Geometry check sheet. Reference: the model listing, model coordinates, mm. A direction names the side the tool comes from. Give positions to 0.01 mm unless a question says otherwise; leave off trailing zeros. Write each loop counter-clockwise with the first axis right and the second up, starting at its lowest first coordinate (ties: lowest second). Pieces come first, ordered by that corner, then holes. Notation, with made-up numbers: M 82,77.5 L 116,77.5 A14 cw 116,91.5 Z; hole C -30.5,36 d7. An arc over 180 degrees is marked long. Write each question's results on one line, items separated by ' | '.
Autodesk Inventor part; units mm, degrees
ref_plane "YZ Plane" through (0, 0, 0) normal (1, 0, 0) x (0, 1, 0)
ref_plane "XZ Plane" through (0, 0, 0) normal (0, 1, 0) x (-1, 0, 0)
ref_plane "XY Plane" through (0, 0, 0) normal (0, 0, 1) x (1, 0, 0)
sketch "Sketch2" plane through (0, 0, 0) normal (0, 0, 1) x (1, 0, 0)
  line L0 (1.5, 7.5) -> (1.5, 10.5)
  line L1 (1.5, 10.5) -> (3, 10.5)
  line L2 (3, 10.5) -> (3, 12.5)
  line L3 (3, 12.5) -> (5.75, 12.5)
  line L4 (5.75, 12.5) -> (10, 7.5)
  line L5 (10, 7.5) -> (10, 0)
  line L6 (1.5, 7.5) -> (5.75, 7.5)
  line L7 (5.75, 7.5) -> (5.75, 0)
  line L8 (5.75, 0) -> (10, 0)
  line L9 (0, 0) -> (0, 19.425)
  dimension "d0" = 6
  dimension "d1" = 3
  dimension "d2" = 11.5
  dimension "d3" = 20
  dimension "d4" = 7.5
  dimension "d5" = 3
  dimension "d6" = 2
revolve "Revolution1" add sketch "Sketch2" angle 360 about axis through (0, 0, 0) along (0, 1, 0)
sketch "Sketch3" plane through (0, 12.5, 0) normal (0, 1, 0) x (1, 0, 0)
  point P0 (0, 0)
  point P1 (0, 7.75)
  dimension "d8" = 7.75
hole "Hole1" at (0, 12.5, -7.75) direction (0, -1, 0) diameter 2.9 end through all counterbore diameter 5.5 counterbore depth 3.5
pattern_circular "Circular Pattern1" count 3 over 360 about axis through (0, -10, 0) along (0, 1, 0) of "Hole1"
properties part number "902-4250 magnet hold"
Q1. Depth check by flat-ended pin: P1, Ø3, axis at y = 4, z = 7.5, coming from the +X side; P2, Ø1.5, axis at y = 2, z = -6, coming from the -X side; P3, Ø2, axis at x = -7, y = 10.5, coming from the +Z side. Enter the tip coordinate at first touch or a pass-through.
Answer key:
P1: stops at x = 8 | P2: stops at x = -8.51 | P3: stops at z = 1.36
Q2. Release check for a two-part mould opening along Z. For faces 1 (the face through (1.2, 7.5, 1.2)), 2 (the face through (5.557, 12.187, -2.304)), 3 (the face through (5.274, 4.437, 3.686)), 4 (the face through (4.3, 0, 4.3)) record: released by +Z, released by -Z, zero draft, split by the parting line, or undercut.
Answer key:
face 1: undercut | face 2: split by the parting line | face 3: undercut | face 4: zero draft
Q3. Access from +Z, -Z, +X, -X, +Y, -Y to the whole of each face (thin tool, end or side, straight path). Record for faces 5 (the face through (1.3, 10.5, 1.3)), 6 (the face through (-0.75, 3.7, 5.7)), 7 (the face through (-0.06, 4.44, -9.2)).
Answer key:
face 5: +Y | face 6: -Y | face 7: +Y, -Y
Q4. Section check B-B (x = 0). Enter the section's corners in (y, z).
Answer key:
outline: M 0,-10 L 7.5,-10 L 8.44,-9.2 L 0,-9.2 Z; M 0,-6.3 L 9,-6.3 L 9,-5 L 12.5,-5 L 12.5,-3 L 10.5,-3 L 10.5,-1.5 L 7.5,-1.5 L 7.5,-5.75 L 0,-5.75 Z; M 0,5.75 L 7.5,5.75 L 7.5,1.5 L 10.5,1.5 L 10.5,3 L 12.5,3 L 12.5,5.75 L 7.5,10 L 0,10 Z
Q5. Section check C-C (y = 11). Enter the section's corners in (x, z) (3 decimals).
Answer key:
outline: M -6.933,1.134 A7.025 ccw -2.484,-6.571 A2.75 cw 2.484,-6.571 A7.025 ccw 6.933,1.134 A2.75 cw 4.448,5.437 A7.025 ccw -4.448,5.437 A2.75 cw Z; hole C 0,0 d6
Q6. Section check A-A (z = 0). Enter the section's corners in (x, y), then the cut area to 4 significant figures.
Answer key:
outline: M -10,0 L -5.75,0 L -5.75,7.5 L -1.5,7.5 L -1.5,10.5 L -3,10.5 L -3,12.5 L -5.75,12.5 L -10,7.5 Z; M 1.5,7.5 L 5.75,7.5 L 5.75,0 L 10,0 L 10,7.5 L 5.75,12.5 L 3,12.5 L 3,10.5 L 1.5,10.5 Z | area: 121.5 mm2
Q7. Section check D-D (y = 8). Enter the section's corners in (x, z) (3 decimals), then the cut area to 3 significant figures.
Answer key:
outline: C 0,0 d19.15; hole C -6.712,3.875 d2.9; hole C 0,0 d3; hole C 0,-7.75 d2.9; hole C 6.712,3.875 d2.9 | area: 261 mm2
Q8. Material ranges on probe 1 along Z at (x, y) = (0, 7); probe 2 along X at (y, z) = (4.5, -0.25); probe 3 along Z at (x, y) = (0, 11.5), recorded low to high. Write a range as [from, to].
Answer key:
probe 1: z = [-10, -9.2], [-6.3, -5.75], [5.75, 10] | probe 2: x = [-10, -5.74], [5.74, 10] | probe 3: z = [-5, -3], [3, 6.6]
